Job drawing, mm, ordinate dimensions from the low corner. One solid piece. A direction names the side the tool comes from. Round coordinates to 2 decimals unless told otherwise and drop trailing zeros. Loops run counter-clockwise (first coordinate to the right, second up) from the corner with the lowest first, then second, coordinate; pieces in that order, holes last.
1) Band-saw the part on B-B, the plane y = 28. Write the cut outline in (x, z).
2) 3-axis set-ups, long thin cutter, end or side, ignore diameter. For the marked faces 5, 6, 7 and 8: which of +Z, -Z, +X, -X, +Y, -Y reach the whole face in a straight line?
3) Probe line 1 (X direction, y = 28, z = 26); line 2 (Z direction, x = 15, y = 30.85); line 3 (Z direction, x = 9.25, y = 28). List the from-to ranges inside material, lowest first.
4) Drop flat-ended pins along their axis: P1, Ø2.5, axis at x = 7, z = 26, coming from the +Y side; P2, Ø13, axis at x = 9, y = 13, coming from the +Z side; P3, Ø3, axis at x = 10.5, z = 11, coming from the -Y side; P4, Ø1.5, axis at x = 14.5, y = 16.5, coming from the -Z side. Give the stop position or say it passes through.
5) Band-saw the part on C-C, the plane x = 2.25. State how many separate pieces and enclosed holes the cut face has, then the cut area to 3 significant figures.
6) Band-saw the part on D-D, the plane y = 11. Write the cut outline in (x, z), then the cut area to 3 significant figures.
7) Band-saw the part on A-A, the plane x = 6. Write the cut outline in (y, z) (3 decimals).
8) Mould opens along X. For the marked faces 1, 2, 3 and 4 say: +X half, -X half, draft (parallel to the pull), parting line (faces both ways), or undercut.
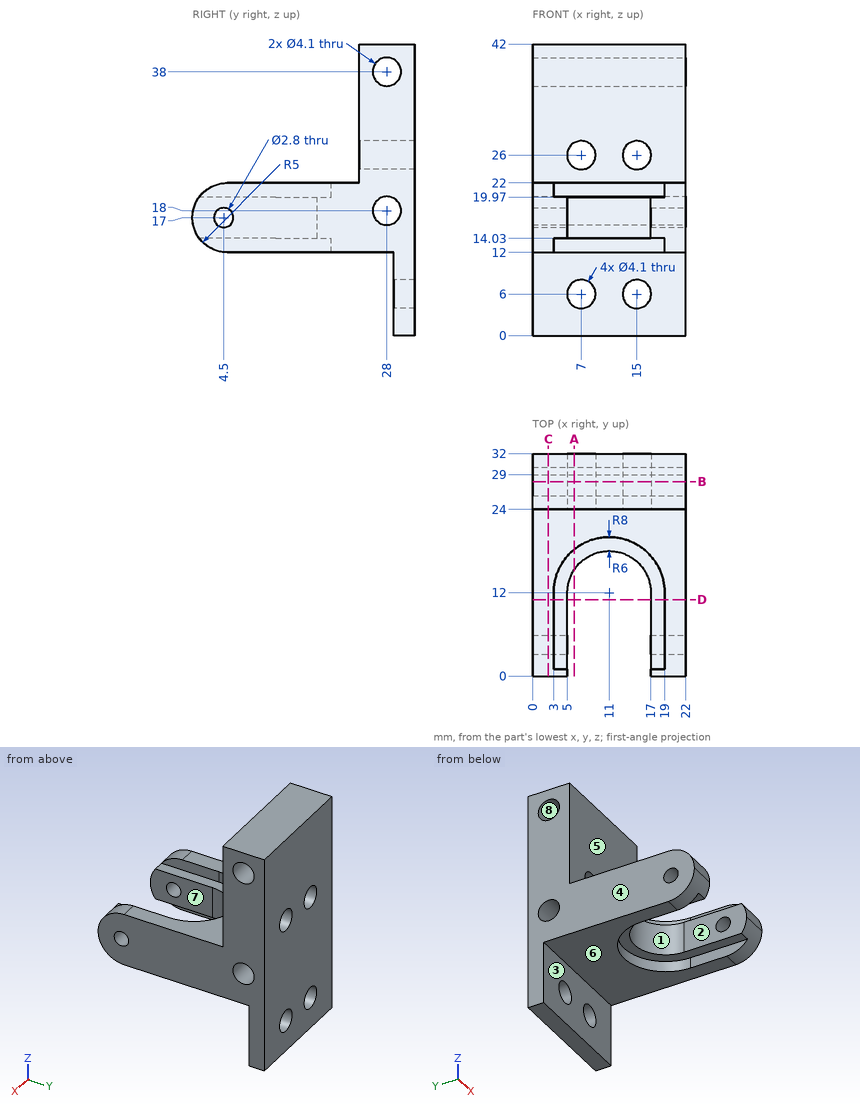
Reported:
1. outline: (0, 12) - (22, 12) - (22, 15.95) - (0, 15.95) - close; (0, 20.05) - (22, 20.05) - (22, 35.95) - (0, 35.95) - close; (0, 40.05) - (22, 40.05) - (22, 42) - (0, 42) - close; hole circle Ø4.1 at (7, 26); hole circle Ø4.1 at (15, 26)
2. face 5: +Z, +X, -X, -Y
2. face 6: -Z, +X, -X, -Y
2. face 7: +Z, -Z, -Y
2. face 8: +X, -X
3. line 1: x = 0 to 4.95, 9.05 to 12.95, 17.05 to 22
3. line 2: z = 0 to 3.95, 8.05 to 23.95, 28.05 to 42
3. line 3: z = 12 to 15.95, 20.05 to 35.95, 40.05 to 42
4. P1: passes through
4. P2: stops at z = 22
4. P3: stops at y = 19.83
4. P4: stops at z = 14.03
5. separate pieces: 1
5. enclosed holes: 3
5. area: 473 mm2
6. outline: (0, 12) - (3, 12) - (3, 14.03) - (5, 14.03) - (5, 19.97) - (3, 19.97) - (3, 22) - (0, 22) - close; (17, 14.03) - (19, 14.03) - (19, 12) - (22, 12) - (22, 22) - (19, 22) - (19, 19.97) - (17, 19.97) - close
6. area: 83.8 mm2
7. outline: (15.317, 14.03) - (18.245, 14.03) - (18.245, 12) - (29, 12) - (29, 7.79) - (32, 7.79) - (32, 24.21) - (24, 24.21) - (24, 22) - (18.245, 22) - (18.245, 19.97) - (15.317, 19.97) - close; (24, 27.79) - (32, 27.79) - (32, 42) - (24, 42) - close; (29, 0) - (32, 0) - (32, 4.21) - (29, 4.21) - close; hole circle Ø4.1 at (28, 18); hole circle Ø4.1 at (28, 38)
8. face 1: undercut
8. face 2: undercut
8. face 3: draft
8. face 4: -X half
